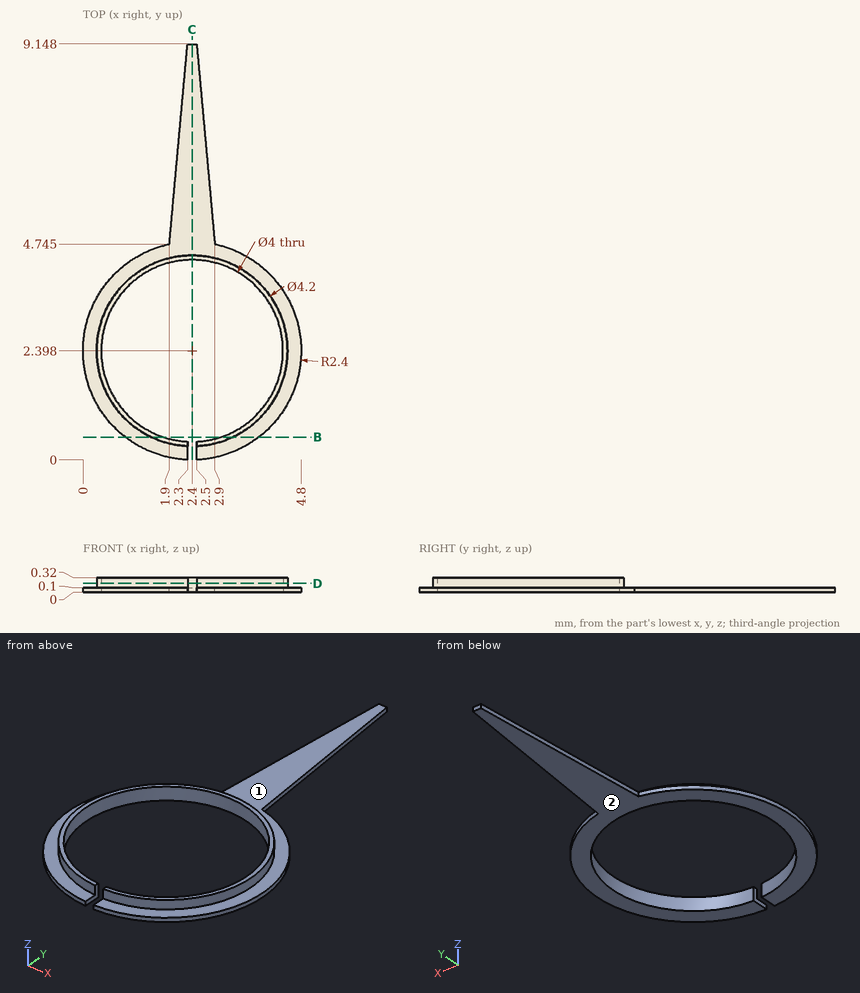
Geometry check sheet. Reference: drawing and pictorial views, mm from the part's lowest x, y, z. A direction names the side the tool comes from. Give positions to 0.01 mm unless a question says otherwise; leave off trailing zeros. Loops run counter-clockwise (first coordinate to the right, second up) from the corner with the lowest first, then second, coordinate; pieces in that order, holes last. Notation, with made-up numbers: M 62,69.5 L 99,69.5 A17 cw 99,92.5 Z; hole C -37.75,4.25 d3. An arc over 180 degrees is marked long. Use a Markdown table: item, result. Add a question column.
Q1. Scan line: line 1 along Y through (x, z) = (4.5, 0.05) (1 decimal). Record every from-to range of solid material in increasing order. Write a range as [from, to].
Q2. Sectioned sample at C-C, the plane x = 2.4. Record the cut outline in (y, z).
Q3. Tool access check on the marked faces 1 and 2. Record the directions out of +Z, -Z, +X, -X, +Y, -Y that give a thin tool (end or side, any length) a straight path to the whole face; none if there is none.
Q4. Sectioned sample at D-D, the plane z = 0.2. Record the cut outline in (x, y).
Q5. Sectioned sample at B-B, the plane y = 0.5. Record the cut outline in (x, z).
Verdict:
| question | item | result |
|---|---|---|
| 1 | line 1 | [1.2, 3.6] |
| 2 | outline | M 4.4,0 L 9.15,0 L 9.15,0.1 L 4.5,0.1 L 4.5,0.32 L 4.4,0.32 Z |
| 3 | face 1 | +Z |
| 3 | face 2 | -Z, +X, -X, +Y, -Y |
| 4 | outline | M 2.3,0.3 L 2.3,0.4 A2 cw long 2.5,0.4 L 2.5,0.3 A2.1 ccw long Z |
| 5 | outline | M 0.93,0 L 1.77,0 L 1.77,0.32 L 1.5,0.32 L 1.5,0.1 L 0.93,0.1 Z; M 3.03,0 L 3.87,0 L 3.87,0.1 L 3.3,0.1 L 3.3,0.32 L 3.03,0.32 Z |
